Autodesk Inventor part; units mm, degrees
ref_plane "YZ Plane" through (0, 0, 0) normal (1, 0, 0) x (0, 1, 0)
ref_plane "XZ Plane" through (0, 0, 0) normal (0, 1, 0) x (-1, 0, 0)
ref_plane "XY Plane" through (0, 0, 0) normal (0, 0, 1) x (1, 0, 0)
sketch "Sketch1" plane through (0, 0, 0) normal (0, 1, 0) x (-1, 0, 0)
  line L0 (0, 0) -> (43, 0)
  line L1 (43, 0) -> (43, -61)
  line L2 (43, -61) -> (0, -61)
  line L3 (0, -61) -> (0, 0)
  dimension "d0" = 61
  dimension "d1" = 43
extrude "Extrusion1" add sketch "Sketch1" along normal blind 10
sketch "Sketch2" plane through (0, 0, 0) normal (1, 0, 0) x (0, 0, -1)
  line L0 (0, 0) -> (0, 10)
  line L1 (0, 5) -> (12.5, 5)
  circle A0 centre (12.5, 5) radius 1.25
  line L2 (0, 10) -> (61, 10)
  line L3 (30.5, 10) -> (30.5, 0)
  circle A1 centre (48.5, 5) radius 1.25
  dimension "d4" = 12.5
  dimension "d5" = 2.5
extrude "Extrusion2" cut sketch "Sketch2" against normal blind 5
sketch "Sketch3" plane through (-43, 0, -61) normal (-1, 0, 0) x (0, 0, 1)
  line L0 (61, 0) -> (0, 0)
  line L1 (61, 0) -> (61, 10)
  line L2 (0, 10) -> (61, 10)
  line L3 (0, 0) -> (0, 10)
  circle A0 centre (48.5, 5) radius 1.25
  circle A1 centre (12.5, 5) radius 1.25
extrude "Extrusion3" cut sketch "Sketch3" against normal blind 5 contours A0 | A1
sketch "Sketch4" plane through (0, 10, 0) normal (0, 1, 0) x (1, 0, 0)
  line L0 (-43, 0) -> (0, 0)
  line L1 (0, 61) -> (-43, 61)
  line L2 (-21.5, 0) -> (-21.5, 6.35)
  line L3 (-21.5, 61) -> (-21.5, 54.65)
  circle A0 centre (-21.5, 6.35) radius 1.25
  circle A1 centre (-21.5, 54.65) radius 1.25
  dimension "d10" = 6.35
  dimension "d11" = 6.35
  dimension "d12" = 2.5
  dimension "d13" = 2.5
extrude "Extrusion4" cut sketch "Sketch4" against normal up to surface (10 mm away)
sketch "Sketch5" plane through (0, 10, 0) normal (0, 1, 0) x (1, 0, 0)
  circle A0 centre (-21.5, 6.35) radius 1.25
  circle A1 centre (-21.5, 54.65) radius 1.25
  line L0 (-43, 0) -> (0, 0)
  line L1 (0, 0) -> (0, 61)
  line L2 (0, 61) -> (-43, 61)
  line L3 (-43, 61) -> (-43, 0)
  line L4 (-8.8, 11.45) -> (-34.2, 11.45)
  line L5 (-34.2, 11.45) -> (-34.2, 49.55)
  line L6 (-34.2, 49.55) -> (-8.8, 49.55)
  line L7 (-8.8, 49.55) -> (-8.8, 11.45)
  line L8 (-8.8, 11.45) -> (-34.2, 49.55) construction
  line L9 (-34.2, 11.45) -> (-8.8, 49.55) construction
  point P0 (-21.5, 30.5)
  dimension "d16" = 25.4
  dimension "d17" = 38.1
extrude "Extrusion5" cut sketch "Sketch5" against normal up to surface (10 mm away) contours L4 L5 L6 L7
sketch "Sketch6" plane through (0, 0, 0) normal (1, 0, 0) x (0, 0, -1)
  line L0 (0, 0) -> (0, 10)
  line L1 (61, 0) -> (0, 0)
  line L2 (0, 10) -> (15.875, 10)
  line L3 (15.875, 10) -> (15.875, 0)
  line L4 (15.875, 0) -> (0, 0)
  line L5 (0, 0) -> (0, 10)
  circle A0 centre (12.5, 5) radius 1.25
  circle A1 centre (48.5, 5) radius 1.25
  line L6 (61, 0) -> (0, 0)
  line L7 (61, 0) -> (61, 10)
  line L8 (0, 10) -> (61, 10)
  line L9 (0, 0) -> (0, 10)
  dimension "d20" = 15.875
extrude "Extrusion6" cut sketch "Sketch6" against normal up to surface (43 mm away) contours L3 L8 L7 L1 | A1
sketch "Sketch7" plane through (0, 10, 0) normal (0, 1, 0) x (1, 0, 0)
  line L0 (-34.2, 15.875) -> (-43, 15.875)
  line L1 (-43, 15.875) -> (-43, 0)
  line L2 (-43, 0) -> (0, 0)
  line L3 (0, 0) -> (0, 15.875)
  line L4 (0, 15.875) -> (-8.8, 15.875)
  line L5 (-8.8, 15.875) -> (-8.8, 11.45)
  line L6 (-8.8, 11.45) -> (-34.2, 11.45)
  line L7 (-34.2, 11.45) -> (-34.2, 15.875)
  circle A0 centre (-21.5, 6.35) radius 1.25
  line L8 (-43, 0) -> (0, 0)
  line L9 (-21.5, 0) -> (-34.2, 0)
  line L10 (-34.2, 0) -> (-34.2, 6.6802)
  circle A1 centre (-34.2, 6.6802) radius 1.5875
  line L11 (-21.5, 0) -> (-21.5, 3.1877)
  circle A2 centre (-8.8, 6.6802) radius 1.5875
  dimension "d23" = 12.7
  dimension "d24" = 6.6802
  dimension "d25" = 3.175
extrude "Extrusion7" cut sketch "Sketch7" against normal blind 25.4 contours A1 | A2
sketch "Sketch8" plane through (0, 0, -15.875) normal (0, 0, -1) x (-1, 0, 0)
  line L0 (34.2, 0) -> (8.8, 0)
  line L1 (8.8, 10) -> (34.2, 10)
  line L2 (8.8, 10) -> (8.8, 0)
  line L3 (0, 0) -> (43, 0)
  line L4 (8.8, 10) -> (15.15, 10)
  line L5 (15.15, 10) -> (15.15, 0)
  line L6 (15.15, 0) -> (8.8, 0)
  line L7 (8.8, 0) -> (8.8, 10)
  circle A0 centre (15.15, 5) radius 1.5875
  line L8 (34.2, 10) -> (27.85, 10)
  line L9 (27.85, 10) -> (27.85, 0)
  line L10 (27.85, 0) -> (34.2, 0)
  line L11 (34.2, 0) -> (34.2, 10)
  circle A1 centre (27.85, 5) radius 1.5875
  line L12 (34.2, 10) -> (34.2, 0)
  line L13 (8.8, 10) -> (8.8, 0)
  dimension "d28" = 6.35
  dimension "d29" = 3.175
  dimension "d30" = 6.35
  dimension "d31" = 3.175
extrude "Extrusion8" cut sketch "Sketch8" against normal up to surface (15.875 mm away) contours A1 L9 | L9 A1 | A0 L5 | L5 A0
properties part number "exBase"
Check sheet for the modelled part. Datum: model origin and axes. Units: mm. A direction names the side the tool comes from. Give positions to 0.01 mm unless a question says otherwise; leave off trailing zeros. Write each loop counter-clockwise with the first axis right and the second up, starting at its lowest first coordinate (ties: lowest second). Pieces come first, ordered by that corner, then holes. Notation, with made-up numbers: (-39, -28) - (14, -28) arc R27 cw to (14, 3) - close; hole circle Ø7 at (-31, -20). An arc over 180 degrees is marked (long way). Answer as a JSON object with one key per item and string values. Group by question number.
1) Access from +Z, -Z, +X, -X, +Y, -Y to the whole of each face (thin tool, end or side, straight path). Record for faces 4 (the face through (-40.53, 4.24, -13.49)), 5 (the face through (-2.46, 3.78, -12.23)), 6 (the face through (-21, 5, -11.45)), 7 (the face through (-21, 10, -8)).
2) Sectioned sample at A-A (z = -12.5). Record the cut outline in (x, y), then the cut area to 3 significant figures.
3) Sectioned sample at C-C (x = -21.5). Record the cut outline in (y, z), then the cut area to 3 significant figures.
4) Sectioned sample at B-B (y = 4.25). Give the number of separate pieces and of enclosed holes in the cut face, then the cut area to 3 significant figures.
5) Depth check by flat-ended pin: P1, Ø3, axis at x = -24, y = 5, coming from the -Z side; P2, Ø0.8, axis at y = 4.5, z = -13, coming from the +X side. Enter the tip coordinate at first touch or a pass-through.
6) Thickness scan on probe 1 along Y at (x, z) = (-39, -12.5); probe 2 along Y at (x, z) = (-27.85, -5); probe 3 along X at (y, z) = (8.75, -14). Record the ranges inside material, lowest first. Write a range as from..to.
7) Release check for a two-part mould opening along Y. For faces 1 (the face through (-21, 0, -8)), 2 (the face through (-21, 5, 0)), 3 (the face through (-5, 5, -12)) record: pulls with the +Y half, pulls with the -Y half, needs draft (parallel to the pull), parting line crosses it, or undercut.
Geometry results:
{
 "1": {"face 4": "-X", "face 5": "+X", "face 6": "-Z, +Y, -Y", "face 7": "+Z, -Z, +X, -X, +Y"},
 "2": {"outline": "(-43, 0) - (-34.2, 0) - (-34.2, 10) - (-43, 10) - (-43, 6.25) - (-38, 6.25) - (-38, 3.75) - (-43, 3.75) - close; (-8.8, 0) - (0, 0) - (0, 3.75) - (-5, 3.75) - (-5, 6.25) - (0, 6.25) - (0, 10) - (-8.8, 10) - close", "area": "151 mm^2"},
 "3": {"outline": "(0, -11.45) - (10, -11.45) - (10, -7.6) - (0, -7.6) - close; (0, -5.1) - (10, -5.1) - (10, 0) - (0, 0) - close", "area": "89.5 mm^2"},
 "4": {"separate pieces": "3", "enclosed holes": "3", "area": "465 mm^2"},
 "5": {"P1": "stops at z = -11.45", "P2": "stops at x = -5"},
 "6": {"probe 1": "y = 0..3.75, 6.25..10", "probe 2": "y = 0..3.41, 6.59..10", "probe 3": "x = -43..-34.2, -8.8..0"},
 "7": {"face 1": "pulls with the -Y half", "face 2": "needs draft", "face 3": "undercut"}
}
